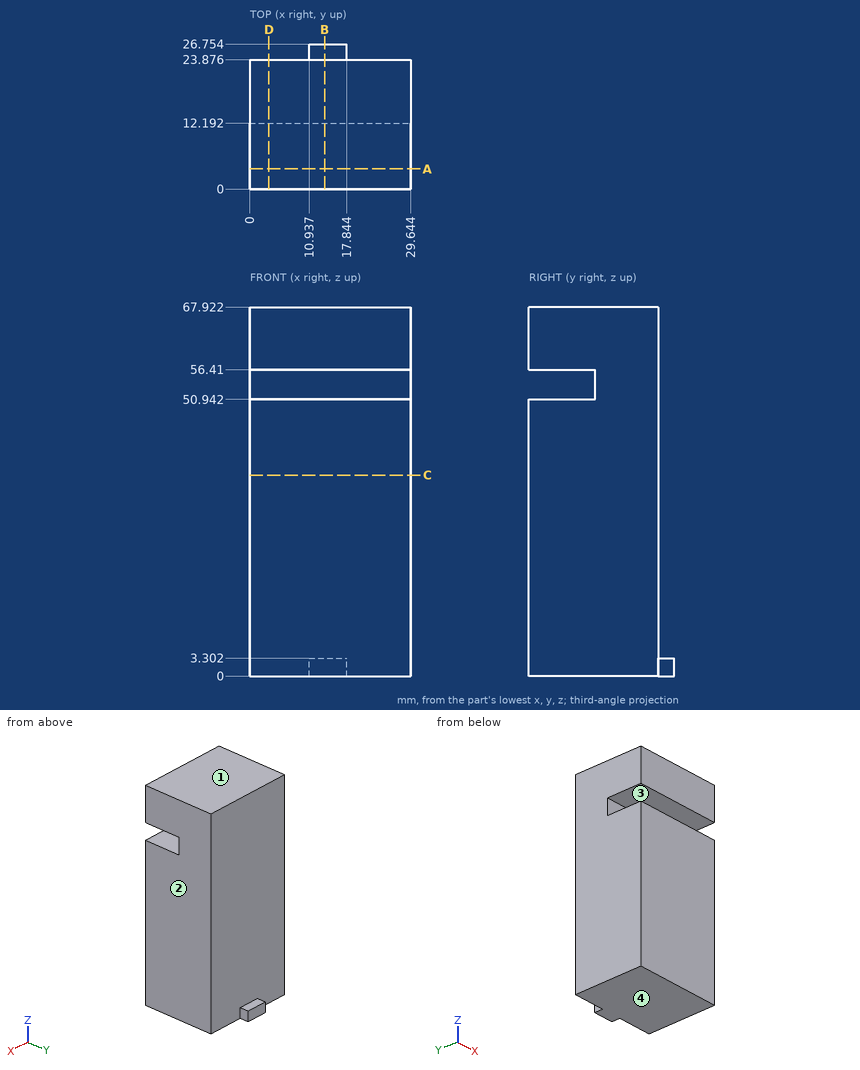
Geometry check sheet. Reference: drawing and pictorial views, mm from the part's lowest x, y, z. Coordinates: 2 decimals unless noted, no trailing zeros. Write each loop counter-clockwise with the first axis right and the second up, starting at its lowest first coordinate (ties: lowest second). Pieces come first, ordered by that corner, then holes. Notation, with made-up numbers: (-30.5, 40) - (8.5, 40) arc R16 cw to (8.5, 58) - close; hole circle Ø11 at (67.5, -24). An arc over 180 degrees is marked (long way). One line per question, with ' | ' between items. Start each with the question number.
1. Section check C-C (z = 37). Enter the section's corners in (x, y).
2. Section check D-D (x = 3.5). Enter the section's corners in (y, z).
3. Draft check along Z on the marked faces 1, 2, 3 and 4. Enter one of: released by +Z, released by -Z, zero draft, split by the parting line, or undercut.
4. Material ranges on line 1 along Z through (x, y) = (5, 4); line 2 along Y through (x, z) = (19, 7), recorded low to high.
5. Section check A-A (y = 3.75). Enter the section's corners in (x, z).
6. Gauge pin test, flat ends, axial feed: P1, Ø0.9, axis at x = 13, y = 25, coming from the +Z side; P2, Ø6, axis at x = 26, z = 10.5, coming from the +Y side; P3, Ø1.4, axis at y = 25, z = 2, coming from the +X side. Record the tip position at first contact, or that the pin passes through.
7. Section check B-B (x = 13.75). Enter the section's corners in (y, z).
Computed values:
1) outline: (0, 0) - (29.64, 0) - (29.64, 23.88) - (0, 23.88) - close
2) outline: (0, 0) - (23.88, 0) - (23.88, 67.92) - (0, 67.92) - (0, 56.41) - (12.19, 56.41) - (12.19, 50.94) - (0, 50.94) - close
3) face 1: released by +Z | face 2: zero draft | face 3: undercut | face 4: released by -Z
4) line 1: 0 to 50.94, 56.41 to 67.92 | line 2: 0 to 23.88
5) outline: (0, 0) - (29.64, 0) - (29.64, 50.94) - (0, 50.94) - close; (0, 56.41) - (29.64, 56.41) - (29.64, 67.92) - (0, 67.92) - close
6) P1: z = 3.3 | P2: y = 23.88 | P3: x = 17.84
7) outline: (0, 0) - (26.75, 0) - (26.75, 3.3) - (23.88, 3.3) - (23.88, 67.92) - (0, 67.92) - (0, 56.41) - (12.19, 56.41) - (12.19, 50.94) - (0, 50.94) - close
